from build123d import *

# Parameters (mm, degrees)
SKETCH1_W           = 20
SKETCH1_H           = 20
BOSS_EXTRUDE2_DEPTH = 2
BOSS_EXTRUDE3_DEPTH = 2


with BuildPart() as part:
    # Sketch1 → Boss-Extrude2 (new body)
    with BuildSketch(Plane(origin=(0, 0, 0), x_dir=(1, 0, 0), z_dir=(0, 1, 0))):
        Rectangle(SKETCH1_W, SKETCH1_H)
    extrude(amount=-BOSS_EXTRUDE2_DEPTH)

    # Sketch2 → Boss-Extrude3 (add)
    with BuildSketch(Plane(origin=(0, 0, 0), x_dir=(1, 0, 0), z_dir=(0, 1, 0))):
        with BuildLine():
            Line((-6, 8), (10, 8))
            Line((10, 8), (10, 10))
            Line((10, 10), (-10, 10))
            Line((-10, 10), (-10, -10))
            Line((-10, -10), (-8, -10))
            Line((-8, -10), (-8, 6))
            ThreePointArc((-8, 6), (-7.414213562, 7.414213562), (-6, 8))
        make_face()
    extrude(amount=BOSS_EXTRUDE3_DEPTH)


solid = part.part
Verification items for the finished model (mm, model axes). A direction names the side the tool comes from. Give positions to 0.01 mm unless a question says otherwise; leave off trailing zeros. Write each loop counter-clockwise with the first axis right and the second up, starting at its lowest first coordinate (ties: lowest second). Pieces come first, ordered by that corner, then holes. Notation, with made-up numbers: M 37,-11 L 56,-11 A17 cw 56,11 Z; hole C 12.5,72.5 d4. An arc over 180 degrees is marked long. Put each result on its own line as item: value. Start each with the question number.
1. Section check C-C (z = 4). Record the cut outline in (x, y), and give its area (3 significant figures).
2. Scan lines: line 1 along Y through (x, z) = (4, 5.25); line 2 along X through (y, z) = (0.9, 5.5). Record each from-to range of solid material in increasing order. Write a range as [from, to].
3. Draft check along X on faces 1 (the face through (0, 0, -10)), 2 (the face through (-7.43, 0.99, -7.4)), 3 (the face through (-10, 0, 0)). Enter one of: +X half, -X half, draft (parallel to the pull), parting line (faces both ways), or undercut.
4. Set-up check for faces 4 (the face through (0, -2, 0)), 5 (the face through (-8, 1, 2)): record each of +Z, -Z, +X, -X, +Y, -Y from which the full face is reachable in a straight line by a thin tool's end or side.
5. Section check A-A (y = 1.2). Record the cut outline in (x, z), and give its area (3 significant figures).
6. Section check B-B (x = 3). Record the cut outline in (y, z).
7. Go/stop test with flat-tipped pins: pin 1 Ø5 at (x, z) = (-4, -2) entering from +Y; pin 2 Ø1 at (y, z) = (1.5, 4) entering from +X; pin 3 Ø2 at (x, y) = (2.5, 1.5) entering from +Z. Record where each tip stops, or that it passes through.
Answer list:
1. outline: M -10,-2 L 10,-2 L 10,0 L -8,0 L -8,2 L -10,2 Z
1. area: 44.0 mm2
2. line 1: [-2, 0]
2. line 2: [-10, -8]
3. face 1: draft
3. face 2: +X half
3. face 3: -X half
4. face 4: +Z, -Z, +X, -X, -Y
4. face 5: +Z, +X, +Y
5. outline: M -10,-10 L 10,-10 L 10,-8 L -6,-8 A2 cw -8,-6 L -8,10 L -10,10 Z
5. area: 76.9 mm2
6. outline: M -2,-10 L 2,-10 L 2,-8 L 0,-8 L 0,10 L -2,10 Z
7. pin 1: y = 0
7. pin 2: x = -8
7. pin 3: z = -8
